Geometry check sheet. Reference: drawing and pictorial views, mm from the part's lowest x, y, z. A direction names the side the tool comes from. Give positions to 0.01 mm unless a question says otherwise; leave off trailing zeros. Order: outer loops, then holes, each group sorted by start corner. A loop starts at its lowest first (then second) coordinate and runs counter-clockwise, first axis right, second up.
Item 1: Access from +Z, -Z, +X, -X, +Y, -Y to the whole of each face (thin tool, end or side, straight path). Record for the marked faces 1 and 2.
Item 2: Material ranges on line 1 along Y through (x, z) = (6.5, 8) (1 decimal); line 2 along X through (y, z) = (5.5, 26.5) (1 decimal); line 3 along Z through (x, y) = (31.5, 10) (1 decimal), recorded low to high.
Item 3: Sectioned sample at B-B on z = 31.5. Record the boundary of the cut face in (x, y) (1 decimal).
Item 4: Gauge pin test, flat end, axial feed: P1, Ø4, axis at y = 6, z = 9, coming from the -X side. Record the tip position at first contact, or that the pin passes through.
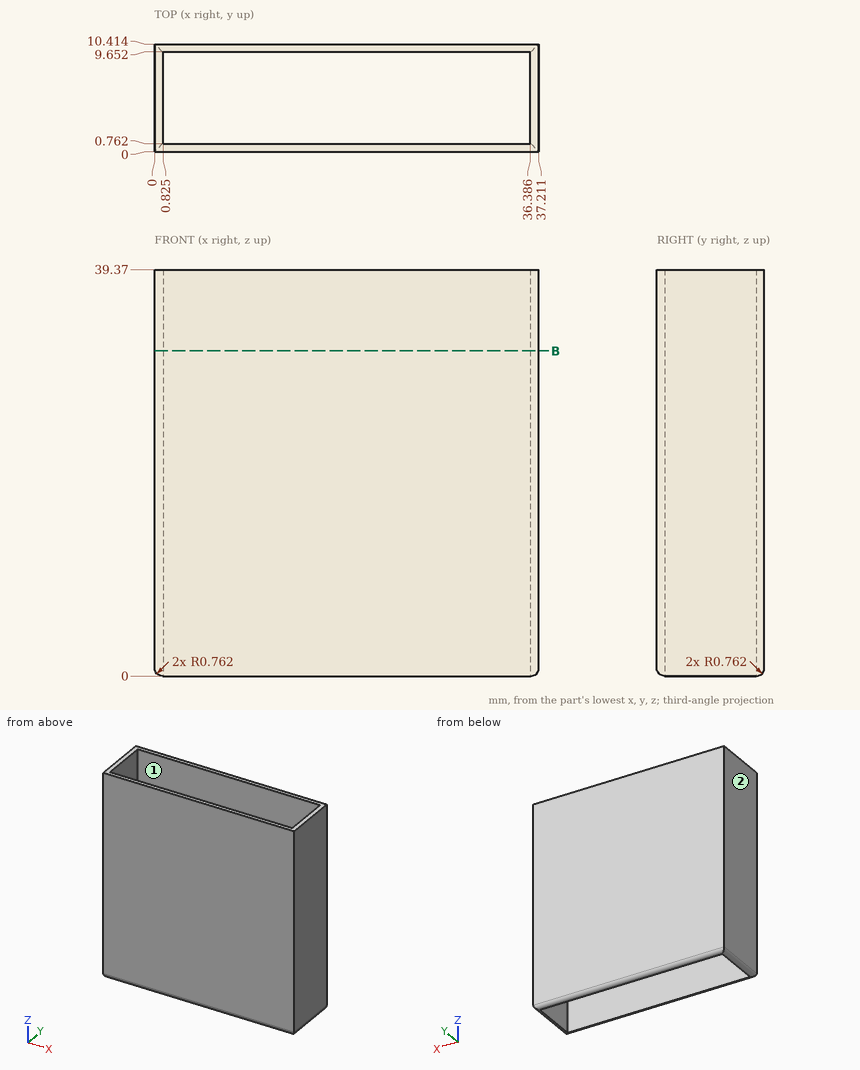
Report:
1. face 1: +Z, -Z
1. face 2: +Z, -Z, -X, +Y, -Y
2. line 1: y = 0 to 0.8, 9.7 to 10.4
2. line 2: x = 0 to 0.8, 36.4 to 37.2
2. line 3: z = 0.1 to 39.4
3. outline: (0, 0) - (37.2, 0) - (37.2, 10.4) - (0, 10.4) - close; hole (0.8, 0.8) - (36.4, 0.8) - (36.4, 9.7) - (0.8, 9.7) - close
4. P1: stops at x = 0
